```python
from build123d import *

# Parameters (mm, degrees)
F0_W           = 95.25
F0_H           = 45.72
F1_DEPTH       = 5.08
F2_W           = 2.54
F2_H           = 45.72
F3_DEPTH       = 25.4
F5_DEPTH       = 95.251
F5_DEPTH_BACK  = 163
F8_W           = 71.12
F8_H           = 31.75
F9_DEPTH       = 22.86
F9_DEPTH_BACK  = 22.86
F10_W          = 66.04
F10_H          = 38.1
F11_DEPTH      = 95.251
F11_DEPTH_BACK = 13.589
F13_DEPTH      = 45.721
F13_DEPTH_BACK = 190
F14_R          = 1.6
F14_R_2        = 13
F15_DEPTH      = 19.305
F16_R          = 5.08


# Not quite as in the source:
# - an extrude ends at something that could not be found from the text; its depth is read off the source's solid


with BuildPart() as f1:
    # F0 (on Right) → F1 (new body)
    with BuildSketch(Plane.YZ):
        with Locations((47.625, -22.86)):
            Rectangle(F0_W, F0_H)
    extrude(amount=F1_DEPTH)

    # F2 (on Right) → F3 (join)
    with BuildSketch(Plane.YZ):
        with Locations((93.98, -22.86)):
            Rectangle(F2_W, F2_H)
        with Locations((1.27, -22.86)):
            Rectangle(F2_W, F2_H)
    extrude(amount=-F3_DEPTH)

    # F4 (on Front) → F5 (cut, two sides)
    with BuildSketch(Plane.XZ) as f5_sk:
        with BuildLine():
            Line((-20.32, -13.97), (-14.605, -13.97))
            ThreePointArc((-14.605, -13.97), (-12.065, -11.43), (-14.605, -8.89))
            Line((-14.605, -8.89), (-20.32, -8.89))
            ThreePointArc((-20.32, -8.89), (-22.86, -11.43), (-20.32, -13.97))
        make_face()
        with BuildLine():
            Line((-20.32, -35.56), (-14.605, -35.56))
            ThreePointArc((-14.605, -35.56), (-12.065, -33.02), (-14.605, -30.48))
            Line((-14.605, -30.48), (-20.32, -30.48))
            ThreePointArc((-20.32, -30.48), (-22.86, -33.02), (-20.32, -35.56))
        make_face()
    extrude(amount=-F5_DEPTH, mode=Mode.SUBTRACT)
    extrude(f5_sk.sketch, amount=F5_DEPTH_BACK, mode=Mode.SUBTRACT)

    # F8 (on plane+point) → F9 (join, two sides)
    with BuildSketch(Plane.XY.offset(-22.86)) as f9_sk:
        with Locations((35.56, -3.429)):
            Rectangle(F8_W, F8_H)
    extrude(amount=-F9_DEPTH)
    extrude(f9_sk.sketch, amount=F9_DEPTH_BACK)

    # F10 (on Front) → F11 (cut, two sides)
    with BuildSketch(Plane.XZ) as f11_sk:
        with Locations((38.1, -22.86)):
            Rectangle(F10_W, F10_H)
    extrude(amount=-F11_DEPTH, mode=Mode.SUBTRACT)
    extrude(f11_sk.sketch, amount=F11_DEPTH_BACK, mode=Mode.SUBTRACT)

    # F12 (on Top) → F13 (cut, two sides)
    with BuildSketch(Plane.XY) as f13_sk:
        Polygon((5.08, 12.446), (71.12, -13.589), (71.12, 12.446), align=None)
    extrude(amount=-F13_DEPTH, mode=Mode.SUBTRACT)
    extrude(f13_sk.sketch, amount=F13_DEPTH_BACK, mode=Mode.SUBTRACT)

    # F14 (on Front) → F15 (cut, through all)
    with BuildSketch(Plane.XZ):
        with Locations((39.37, -7.36)):
            Circle(F14_R)
        with Locations((25.9466062413, -15.11)):
            Circle(F14_R)
        with Locations((25.9466062413, -30.61)):
            Circle(F14_R)
        with Locations((39.37, -38.36)):
            Circle(F14_R)
        with Locations((52.7933937587, -30.61)):
            Circle(F14_R)
        with Locations((52.7933937587, -15.11)):
            Circle(F14_R)
        with Locations((39.37, -22.86)):
            Circle(F14_R_2)
    extrude(amount=F15_DEPTH, mode=Mode.SUBTRACT)

    # F16
    f16_edges = [f1.edges().sort_by_distance(p)[0] for p in [
        (0, 92.71, -22.86),
        (0, 2.54, -22.86),
        (0, 0, -22.86),
        (0, -19.304, -22.86),
        (5.08, -13.589, -22.86),
        (5.08, -0.5715, -3.81),
        (5.08, -0.5715, -41.91),
        (5.08, 12.446, -1.905),
        (5.08, 12.446, -43.815),
        (5.08, 95.25, -22.86),
    ]]
    fillet(f16_edges, radius=F16_R)


solid = f1.part
```
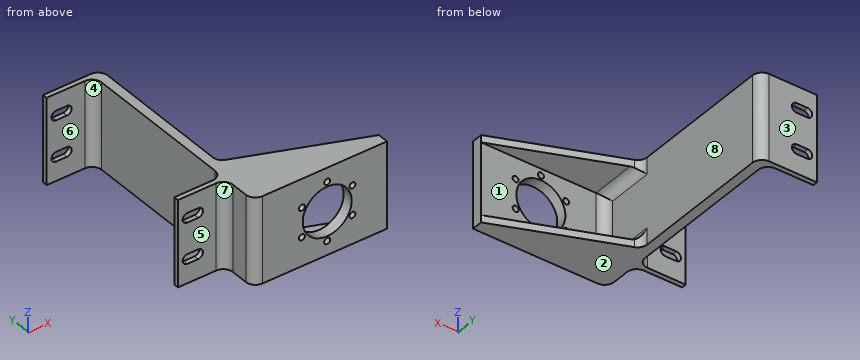
Read the model definition and answer for the solid it produces. Units are mm, in the model's axes. Face numbers are marked on the shaded views. A direction names the side the tool comes from. Round coordinates to 2 decimals unless told otherwise and drop trailing zeros. Loops run counter-clockwise (first coordinate to the right, second up) from the corner with the lowest first, then second, coordinate; pieces in that order, holes last. Notation, with made-up numbers: (58, 89.25) -> (69, 89.25) arc R25 cw to (69, 109.25) -> close; hole circle Ø5 at (-1, -26.75). An arc over 180 degrees is marked (long way). One line per item, written item: value.
1) For the marked faces 1, 2, 3, 4 and 5, determine the directions among +Z, -Z, +X, -X, +Y, -Y from which every point of the face is accessible in a straight line to the end or side of a thin tool.
Answer list:
face 1: +X, +Y
face 2: -Z, +X, -X, +Y, -Y
face 3: +Z, -Z, +X, -X, +Y
face 4: +Z, -Z, -X
face 5: +Z, -Z, -X, -Y
2) A cutting plane is placed at C-C (y = -3.5). Determine the outline of the cut face in (x, z).
Answer list:
outline: (-0.25, -45.72) -> (45.53, -45.72) -> (45.53, -41.91) -> (10.16, -41.91) arc R5.08 cw to (5.08, -36.83) -> (5.08, -8.89) arc R5.08 cw to (10.16, -3.81) -> (45.53, -3.81) -> (45.53, 0) -> (-0.25, 0) -> close
3) A cutting plane is placed at B-B (x = -19). Determine the outline of the cut face in (y, z).
Answer list:
outline: (0, -45.72) -> (2.54, -45.72) -> (2.54, -35.56) -> (0, -35.56) -> close; (0, -30.48) -> (2.54, -30.48) -> (2.54, -13.97) -> (0, -13.97) -> close; (0, -8.89) -> (2.54, -8.89) -> (2.54, 0) -> (0, 0) -> close; (92.71, -45.72) -> (95.25, -45.72) -> (95.25, -35.56) -> (92.71, -35.56) -> close; (92.71, -30.48) -> (95.25, -30.48) -> (95.25, -13.97) -> (92.71, -13.97) -> close; (92.71, -8.89) -> (95.25, -8.89) -> (95.25, 0) -> (92.71, 0) -> close
4) Consider L1, parallel to Z at x = 39.37, y = -18.1; L2, parallel to Y at x = -11, z = -10.5; L3, parallel to X at y = -17.15, z = -15.11. Determine where each line is inside the solid, lowest interval first. Write a range as [from, to].
Answer list:
L1: z = [-45.72, -39.96], [-36.76, -35.86], [-9.86, -8.96], [-5.76, 0]
L2: y = [0, 2.54], [92.71, 95.25]
L3: x = [0.93, 24.35], [27.55, 28.93], [49.81, 51.19], [54.39, 71.12]
5) The mould has two halves that part along Y. Classify the marked faces 6, 7 and 8: pulls with the +Y half, pulls with the -Y half, needs draft (parallel to the pull), parting line crosses it, or undercut.
Answer list:
face 6: undercut
face 7: pulls with the -Y half
face 8: needs draft
6) Flat-ended cylindrical pins translate along their axes: P1, Ø16.5, axis at x = -12, z = -31, coming from the -Y side; P2, Ø2, axis at x = -17.5, y = 93.5, coming from the +Z side; P3, Ø1.5, axis at y = 74.5, z = -18, coming from the +X side; P4, Ø1.9, axis at x = 52.79, z = -15.11, coming from the +Y side. Find the tip coordinate at first contact, or state that the pin passes through.
Answer list:
P1: stops at y = -0.18
P2: stops at z = 0
P3: stops at x = 5.08
P4: passes through
7) A cutting plane is placed at A-A (z = -38.36). Determine the outline of the cut face in (x, y).
Answer list:
outline: (-25.4, 0) -> (-5.08, 0) arc R5.08 cw to (0, -5.08) -> (0, -14.22) arc R5.08 ccw to (5.08, -19.3) -> (37.77, -19.3) -> (37.77, -13.59) -> (10.16, -13.59) arc R5.08 cw to (5.32, -10.04) -> (5.32, 14.37) arc R5.08 cw to (5.08, 15.9) -> (5.08, 90.17) arc R5.08 ccw to (0, 95.25) -> (-25.4, 95.25) -> (-25.4, 92.71) -> (-5.08, 92.71) arc R5.08 cw to (0, 87.63) -> (0, 7.62) arc R5.08 cw to (-5.08, 2.54) -> (-25.4, 2.54) -> close; (40.97, -19.3) -> (71.12, -19.3) -> (71.12, -13.59) -> (40.97, -13.59) -> close
8) A cutting plane is placed at D-D (x = 39.37). Determine the outline of the cut face in (y, z), and give its area (3 significant figures).
Answer list:
outline: (-19.3, -45.72) -> (-1.07, -45.72) -> (-1.07, -41.91) -> (-13.59, -41.91) -> (-13.59, -39.96) -> (-19.3, -39.96) -> close; (-19.3, -36.76) -> (-13.59, -36.76) -> (-13.59, -35.86) -> (-19.3, -35.86) -> close; (-19.3, -9.86) -> (-13.59, -9.86) -> (-13.59, -8.96) -> (-19.3, -8.96) -> close; (-19.3, -5.76) -> (-13.59, -5.76) -> (-13.59, -3.81) -> (-1.07, -3.81) -> (-1.07, 0) -> (-19.3, 0) -> close
area: 172 mm²
